Could you check a few things on this model? Use its own coordinates, in mm. Give positions to 0.01 mm unless a question says otherwise; leave off trailing zeros. Write each loop counter-clockwise with the first axis right and the second up, starting at its lowest first coordinate (ties: lowest second). Pieces come first, ordered by that corner, then holes. Notation, with made-up numbers: (-36.75, -19.75) - (-10.75, -19.75) arc R14 cw to (-10.75, -10.75) - close; hole circle Ø7 at (-8, -18.5). An arc over 180 degrees is marked (long way). Use one line per item in the form item = value.
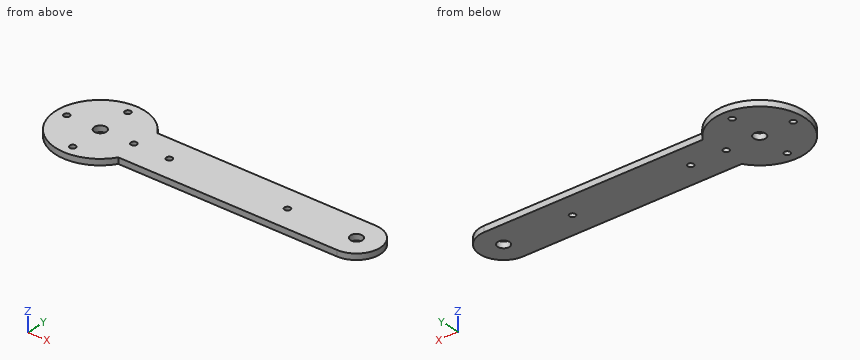
```python
from build123d import *

# Parameters (mm, degrees)
BOSS_EXTRU_1_DEPTH      = 3
ESQUISSE2_R             = 3
ESQUISSE2_R_2           = 1.5
ENL_V_MAT_EXTRU_1_DEPTH = 78.987178433
ESQUISSE3_R             = 22.5
ESQUISSE3_R_2           = 3
BOSS_EXTRU_2_DEPTH      = 3
ESQUISSE4_R             = 1.5
ENL_V_MAT_EXTRU_2_DEPTH = 91.396349484


with BuildPart() as part:
    # Esquisse1 → Boss.-Extru.1 (new body)
    with BuildSketch(Plane.XY):
        with BuildLine():
            Line((-65, 12), (65, 12))
            ThreePointArc((65, 12), (77, 0), (65, -12))
            Line((65, -12), (-65, -12))
            ThreePointArc((-65, -12), (-77, 0), (-65, 12))
        make_face()
    extrude(amount=BOSS_EXTRU_1_DEPTH)

    # Esquisse2 → Enlèv. mat.-Extru.1 (cut, through all)
    with BuildSketch(Plane.XY.offset(3)):
        with Locations((-65, 0)):
            Circle(ESQUISSE2_R)
        with Locations(Location((65, 0, 0), (0, 0, 180))):
            Circle(ESQUISSE2_R)
        with Locations((-30, 0)):
            Circle(ESQUISSE2_R_2)
        with Locations(Location((30, 0, 0), (0, 0, 180))):
            Circle(ESQUISSE2_R_2)
    extrude(amount=-ENL_V_MAT_EXTRU_1_DEPTH, mode=Mode.SUBTRACT)

    # Esquisse3 → Boss.-Extru.2 (add)
    with BuildSketch(Plane.XY.offset(3)):
        with Locations((-65, 0)):
            Circle(ESQUISSE3_R)
        with Locations((-65, 0)):
            Circle(ESQUISSE3_R_2, mode=Mode.SUBTRACT)
    extrude(amount=-BOSS_EXTRU_2_DEPTH)

    # Esquisse4 → Enlèv. mat.-Extru.2 (cut, through all)
    with BuildSketch(Plane(origin=(0, 0, 0), x_dir=(-1, 0, 0), z_dir=(0, 0, -1))):
        with Locations((65, 17)):
            Circle(ESQUISSE4_R)
        with Locations((82, 0)):
            Circle(ESQUISSE4_R)
        with Locations((65, -17)):
            Circle(ESQUISSE4_R)
        with Locations((48, 0)):
            Circle(ESQUISSE4_R)
    extrude(amount=-ENL_V_MAT_EXTRU_2_DEPTH, mode=Mode.SUBTRACT)


solid = part.part
```
1. Imagine slicing it at A-A, the plane z = 1.9. State how many separate pieces and enclosed holes the cut face has, and give its area (3 significant figures).
Response values:
separate_pieces = 1
enclosed_holes = 8
area = 4,320 mm²
2. Imagine slicing it at D-D, the plane x = -82. List the corners of the cut face in (y, z) for me, and give its area (3 significant figures).
Response values:
outline = (-14.74, 0) - (-1.5, 0) - (-1.5, 3) - (-14.74, 3) - close; (1.5, 0) - (14.74, 0) - (14.74, 3) - (1.5, 3) - close
area = 79.4 mm²
3. For pin 1 (1.5 mm diameter, centred on x = 26, y = 5, fed in from -Z); pin 2 (1.5 mm diameter, centred on y = 15, z = 2, fed in from +X); pin 3 (1 mm diameter, centred on x = -3, z = 1, fed in from -Y), each with a flat end and sliding along its axis, tell me the tip position at first contact or that it passes through.
Response values:
pin_1 = 0
pin_2 = -47.59
pin_3 = -12
4. Imagine slicing it at B-B, the plane x = -65. List the corners of the cut face in (y, z) for me.
Response values:
outline = (-22.5, 0) - (-18.5, 0) - (-18.5, 3) - (-22.5, 3) - close; (-15.5, 0) - (-3, 0) - (-3, 3) - (-15.5, 3) - close; (3, 0) - (15.5, 0) - (15.5, 3) - (3, 3) - close; (18.5, 0) - (22.5, 0) - (22.5, 3) - (18.5, 3) - close
5. If I drill on line 1 (Y direction, x = -65, z = 2.05); line 2 (Y direction, x = 30, z = 1.7); line 3 (Y direction, x = 65, z = 1.85), over which ranges is the centre line in solid material (lowest first)? Write a range as from..to.
Response values:
line_1 = -22.5..-18.5, -15.5..-3, 3..15.5, 18.5..22.5
line_2 = -12..-1.5, 1.5..12
line_3 = -12..-3, 3..12
6. Imagine slicing it at C-C, the plane y = 17. List the corners of the cut face in (x, z) for me.
Response values:
outline = (-79.74, 0) - (-66.5, 0) - (-66.5, 3) - (-79.74, 3) - close; (-63.5, 0) - (-50.26, 0) - (-50.26, 3) - (-63.5, 3) - close
